from build123d import *

# Parameters (mm, degrees)
IZIM1_R                     = 190
IZIM1_R_2                   = 7
IZIM1_R_3                   = 18
IZIM1_R_4                   = 5.1
Y_KSEKLIK_EKSTR_ZYON1_DEPTH = 10


with BuildPart() as part:
    # Çizim1 → Yükseklik-Ekstrüzyon1 (new body)
    with BuildSketch(Plane.XY):
        Circle(IZIM1_R)
        with Locations((0, 170)):
            Circle(IZIM1_R_2, mode=Mode.SUBTRACT)
        with Locations((-99.92349289, 137.532889044)):
            Circle(IZIM1_R_2, mode=Mode.SUBTRACT)
        with Locations((-161.67960777, 52.532889044)):
            Circle(IZIM1_R_2, mode=Mode.SUBTRACT)
        with Locations((-161.67960777, -52.532889044)):
            Circle(IZIM1_R_2, mode=Mode.SUBTRACT)
        with Locations((-99.92349289, -137.532889044)):
            Circle(IZIM1_R_2, mode=Mode.SUBTRACT)
        with Locations((0, -170)):
            Circle(IZIM1_R_2, mode=Mode.SUBTRACT)
        with Locations((99.92349289, -137.532889044)):
            Circle(IZIM1_R_2, mode=Mode.SUBTRACT)
        with Locations((161.67960777, -52.532889044)):
            Circle(IZIM1_R_2, mode=Mode.SUBTRACT)
        with Locations((161.67960777, 52.532889044)):
            Circle(IZIM1_R_2, mode=Mode.SUBTRACT)
        with Locations((99.92349289, 137.532889044)):
            Circle(IZIM1_R_2, mode=Mode.SUBTRACT)
        Circle(IZIM1_R_3, mode=Mode.SUBTRACT)
        with Locations((-38.890872965, 38.890872965)):
            Circle(IZIM1_R_4, mode=Mode.SUBTRACT)
        with Locations((38.890872965, 38.890872965)):
            Circle(IZIM1_R_4, mode=Mode.SUBTRACT)
        with Locations((38.890872965, -38.890872965)):
            Circle(IZIM1_R_4, mode=Mode.SUBTRACT)
        with Locations((-38.890872965, -38.890872965)):
            Circle(IZIM1_R_4, mode=Mode.SUBTRACT)
    extrude(amount=Y_KSEKLIK_EKSTR_ZYON1_DEPTH)


solid = part.part
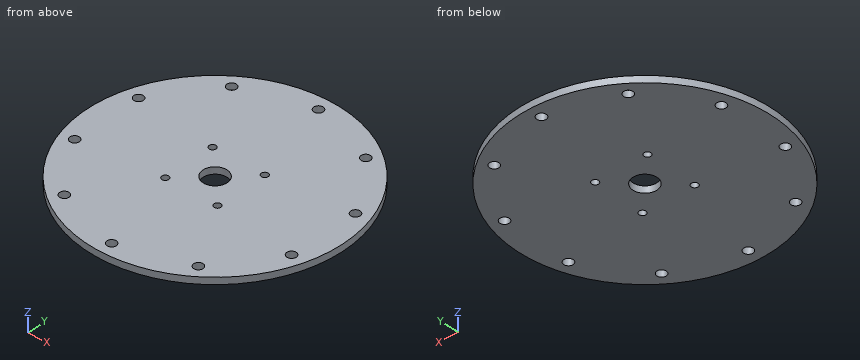
Check sheet for the modelled part. Datum: model origin and axes. Units: mm. Round coordinates to 2 decimals unless told otherwise and drop trailing zeros. Loops run counter-clockwise (first coordinate to the right, second up) from the corner with the lowest first, then second, coordinate; pieces in that order, holes last. Notation, with made-up numbers: (31.5, 73) -> (65.5, 73) arc R13 ccw to (65.5, 79) -> close; hole circle Ø6 at (3.25, 70.5). An arc over 180 degrees is marked (long way). Put each result on its own line as item: value. Start each with the question number.
1. Gauge pin test, flat ends, axial feed: pin 1 (4 mm diameter, centred on y = -55, z = 3.5, fed in from -X); pin 2 (1 mm diameter, centred on y = 31, z = 8, fed in from +X); pin 3 (1.5 mm diameter, centred on y = 82, z = 8.5, fed in from -X); pin 4 (18 mm diameter, centred on x = -161.68, y = 52.53, fed in from -Z). Record the tip position at first contact, or that the pin passes through.
2. Scan lines: probe 1 along Y at (x, z) = (5, 2.75); probe 2 along X at (y, z) = (-35, 6.5); probe 3 along X at (y, z) = (-142, 0.5). Record each from-to range of solid material in increasing order.
3. Section check B-B (x = 0). Enter the section's corners in (y, z).
4. Section check A-A (y = 0). Enter the section's corners in (x, z), plus the area to 3 significant figures.
5. Section check D-D (y = 170). Enter the section's corners in (x, z), plus the area to 3 significant figures.
6. Section check C-C (z = 6.75). Give the number of separate pieces and of enclosed holes in the cut face, plus the area to 3 significant figures.
Findings:
1. pin 1: stops at x = -182.46
1. pin 2: stops at x = 187.54
1. pin 3: stops at x = -171.75
1. pin 4: stops at z = 0
2. probe 1: y = -189.93 to -174.9, -165.1 to -17.29, 17.29 to 165.1, 174.9 to 189.93
2. probe 2: x = -186.75 to -42.19, -35.59 to 35.59, 42.19 to 186.75
2. probe 3: x = -126.24 to -105.31, -94.53 to 94.53, 105.31 to 126.24
3. outline: (-190, 0) -> (-177, 0) -> (-177, 10) -> (-190, 10) -> close; (-163, 0) -> (-18, 0) -> (-18, 10) -> (-163, 10) -> close; (18, 0) -> (163, 0) -> (163, 10) -> (18, 10) -> close; (177, 0) -> (190, 0) -> (190, 10) -> (177, 10) -> close
4. outline: (-190, 0) -> (-18, 0) -> (-18, 10) -> (-190, 10) -> close; (18, 0) -> (190, 0) -> (190, 10) -> (18, 10) -> close
4. area: 3,440 mm^2
5. outline: (-84.85, 0) -> (-7, 0) -> (-7, 10) -> (-84.85, 10) -> close; (7, 0) -> (84.85, 0) -> (84.85, 10) -> (7, 10) -> close
5. area: 1,560 mm^2
6. separate pieces: 1
6. enclosed holes: 15
6. area: 111,000 mm^2
